```python
from build123d import *

# Parameters (mm, degrees)
SKETCH1_R           = 10
BOSS_EXTRUDE1_DEPTH = 15


with BuildPart() as part:
    # Sketch1 → Boss-Extrude1 (new, symmetric)
    with BuildSketch(Plane.XY):
        with BuildLine():
            Line((60, 40), (90, 40))
            Line((90, 40), (90, -20))
            ThreePointArc((90, -20), (84.142135624, -34.142135624), (70, -40))
            Line((70, -40), (60, -40))
            Line((60, -40), (60, -35))
            ThreePointArc((60, -35), (58.535533906, -31.464466094), (55, -30))
            Line((55, -30), (-55, -30))
            ThreePointArc((-55, -30), (-58.535533906, -31.464466094), (-60, -35))
            Line((-60, -35), (-60, -40))
            Line((-60, -40), (-70, -40))
            ThreePointArc((-70, -40), (-84.142135624, -34.142135624), (-90, -20))
            Line((-90, -20), (-90, 40))
            Line((-90, 40), (-60, 40))
            ThreePointArc((-60, 40), (0, -20), (60, 40))
        make_face()
        with Locations((-75.702110111, -20)):
            Circle(SKETCH1_R, mode=Mode.SUBTRACT)
        with Locations((75.7, -20)):
            Circle(SKETCH1_R, mode=Mode.SUBTRACT)
    extrude(amount=BOSS_EXTRUDE1_DEPTH, both=True)


solid = part.part
```
Verification items for the finished model (mm, model axes). A direction names the side the tool comes from. Give positions to 0.01 mm unless a question says otherwise; leave off trailing zeros. Loops run counter-clockwise (first coordinate to the right, second up) from the corner with the lowest first, then second, coordinate; pieces in that order, holes last.
1. Mould release check, pull along Y, two halves, no side actions. Record for faces 1 (the cylindrical face through (-83.986, -34.297, 0.21)), 2 (the flat face through (-90, 10, 0)), 3 (the cylindrical face through (-83.07, -13.24, -0.21)): released by +Y, released by -Y, zero draft, split by the parting line, or undercut.
2. Section check D-D, the plane y = -22. Enter the section's corners in (x, z).
3. Thickness scan on line 1 (X direction, y = -14, z = 11.75); line 2 (X direction, y = -12, z = 13.75); line 3 (X direction, y = -34.5, z = -11.25). Record the ranges inside material, lowest first.
4. Go/stop test with flat-tipped pins: pin 1 Ø6 at (x, z) = (-43.5, 5) entering from +Y; pin 2 Ø12 at (x, z) = (44, 0) entering from +Y; pin 3 Ø3 at (x, z) = (-40.5, -6) entering from -Y. Record where each tip stops, or that it passes through.
5. Set-up check for faces 4 (the flat face through (60, -38, 0)), 5 (the flat face through (21, -17, -15)): record each of +Z, -Z, +X, -X, +Y, -Y from which the full face is reachable in a straight line by a thin tool's end or side.
6. Section check B-B, the plane x = 75.7. Enter the section's corners in (y, z), then the cut area to 3 significant figures.
7. Section check C-C, the plane z = 12.5. Enter the section's corners in (x, y), then the cut area to 3 significant figures.
8. Section check A-A, the plane y = -0.5. Enter the section's corners in (x, z), then the cut area to 3 significant figures.
Geometry says:
1. face 1: released by -Y
1. face 2: zero draft
1. face 3: undercut
2. outline: (-89.9, -15) - (-85.5, -15) - (-85.5, 15) - (-89.9, 15) - close; (-65.9, -15) - (65.9, -15) - (65.9, 15) - (-65.9, 15) - close; (85.5, -15) - (89.9, -15) - (89.9, 15) - (85.5, 15) - close
3. line 1: x = -90 to -83.7, -67.7 to -26.15, 26.15 to 67.7, 83.7 to 90
3. line 2: x = -90 to -81.7, -69.7 to -29.93, 29.93 to 69.7, 81.7 to 90
3. line 3: x = -83.77 to -59.97, 59.97 to 83.77
4. pin 1: stops at y = 2.08
4. pin 2: stops at y = 6.83
4. pin 3: stops at y = -30
5. face 4: +Z, -Z, -Y
5. face 5: -Z, +X, -X, +Y, -Y
6. outline: (-39.17, -15) - (-30, -15) - (-30, 15) - (-39.17, 15) - close; (-10, -15) - (40, -15) - (40, 15) - (-10, 15) - close
6. area: 1,780 mm2
7. outline: (-90, -20) arc R20 ccw to (-70, -40) - (-60, -40) - (-60, -35) arc R5 cw to (-55, -30) - (55, -30) arc R5 cw to (60, -35) - (60, -40) - (70, -40) arc R20 ccw to (90, -20) - (90, 40) - (60, 40) arc R60 cw to (-60, 40) - (-90, 40) - close; hole circle Ø20 at (-75.7, -20); hole circle Ø20 at (75.7, -20)
7. area: 6,760 mm2
8. outline: (-90, -15) - (-44.27, -15) - (-44.27, 15) - (-90, 15) - close; (44.27, -15) - (90, -15) - (90, 15) - (44.27, 15) - close
8. area: 2,740 mm2
